```python
from build123d import *

# Parameters (mm, degrees)
SKETCH_1_R      = 1.1
EXTRUDE_1_DEPTH = 0.6
SKETCH_2_W      = 4.9
SKETCH_2_H      = 3.9
EXTRUDE_2_DEPTH = 1.75


with BuildPart() as part:
    # 草图1 → 凸台-拉伸1 (new body)
    with BuildSketch(Plane(origin=(0, 0, 0), x_dir=(1, 0, 0), z_dir=(0, 1, 0))):
        with BuildLine():
            Line((-4.123105626, 8), (4.123105626, 8))
            ThreePointArc((4.123105626, 8), (6.005155898, 6.703588789), (7.5, 4.974937186))
            Line((7.5, 4.974937186), (7.5, -4.974937186))
            ThreePointArc((7.5, -4.974937186), (6.005155898, -6.703588789), (4.123105626, -8))
            Line((4.123105626, -8), (-4.123105626, -8))
            ThreePointArc((-4.123105626, -8), (-6.005155898, -6.703588789), (-7.5, -4.974937186))
            Line((-7.5, -4.974937186), (-7.5, 4.974937186))
            ThreePointArc((-7.5, 4.974937186), (-6.005155898, 6.703588789), (-4.123105626, 8))
        make_face()
        with Locations((-6, 0)):
            Circle(SKETCH_1_R, mode=Mode.SUBTRACT)
        with Locations((6, 0)):
            Circle(SKETCH_1_R, mode=Mode.SUBTRACT)
    extrude(amount=EXTRUDE_1_DEPTH)

    # 草图2 → 凸台-拉伸2 (add)
    with BuildSketch(Plane(origin=(0, 0.6, 0), x_dir=(1, 0, 0), z_dir=(0, 1, 0))):
        Rectangle(SKETCH_2_W, SKETCH_2_H)
    extrude(amount=EXTRUDE_2_DEPTH)


solid = part.part
```
Source: CAD feature listing. Evaluate the final solid. Frame: model axes, mm. A direction names the side the tool comes from. Coordinates: 2 decimals unless noted, no trailing zeros. Write each loop counter-clockwise with the first axis right and the second up, starting at its lowest first coordinate (ties: lowest second). Pieces come first, ordered by that corner, then holes. Notation, with made-up numbers: (82.25, 85) -> (130.25, 85) arc R13 ccw to (130.25, 108) -> close; hole circle Ø1 at (80.5, -28). An arc over 180 degrees is marked (long way). Return JSON: item names as keys, results as strings. Group by question number.
1) Section query D-D, the plane x = -1.75. Return loops of the section in (y, z).
2) Mould query, pull axis X, two halves, no side actions, for faces 1 (the face through (0, 0, 0)), 2 (the face through (7.016, 0.296, 0.421)), 3 (the face through (-2.45, 1, 0)). Classes: +X half, -X half, draft (parallel to the pull), parting line (faces both ways), or undercut.
3) Section query C-C, the plane y = 0.3. Return loops of the section in (x, z).
4) Section query A-A, the plane z = 0. Return loops of the section in (x, y), plus the area to 3 significant figures.
5) Ray query, line 1 along X through (y, z) = (0.45, 0); line 2 along Y through (x, z) = (-0.5, -5.5); line 3 along Z through (x, y) = (6, 0.3). Return the intervals inside material, ascending.
6) Contact query for flat-ended pins moving along their axis: P1, Ø0.5, axis at x = 1, y = 1.5, coming from the +Z side; P2, Ø2, axis at x = 4.5, z = -3, coming from the +Y side; P3, Ø1, axis at x = 6, y = 1, coming from the +Z side. Output: stop coordinate, or through.
7) Section query B-B, the plane x = -6. Return loops of the section in (y, z), plus the area to 3 significant figures.
8) Set-up query: faces 4 (the face through (2.45, 1, 0)), 5 (the face through (0, 1, 1.95)), 6 (the face through (0, 1, -1.95)). Return all of +Z, -Z, +X, -X, +Y, -Y with unobstructed straight access to the full face (end or side cutting, diameter ignored); none if empty.
From the geometry:
{
 "1": {"outline": "(0, -8) -> (0.6, -8) -> (0.6, -1.95) -> (2.35, -1.95) -> (2.35, 1.95) -> (0.6, 1.95) -> (0.6, 8) -> (0, 8) -> close"},
 "2": {"face 1": "draft", "face 2": "undercut", "face 3": "-X half"},
 "3": {"outline": "(-7.5, -4.97) arc R9 ccw to (-4.12, -8) -> (4.12, -8) arc R9 ccw to (7.5, -4.97) -> (7.5, 4.97) arc R9 ccw to (4.12, 8) -> (-4.12, 8) arc R9 ccw to (-7.5, 4.97) -> close; hole circle Ø2.2 at (-6, 0); hole circle Ø2.2 at (6, 0)"},
 "4": {"outline": "(-7.5, 0) -> (-7.1, 0) -> (-7.1, 0.6) -> (-7.5, 0.6) -> close; (-4.9, 0) -> (4.9, 0) -> (4.9, 0.6) -> (2.45, 0.6) -> (2.45, 2.35) -> (-2.45, 2.35) -> (-2.45, 0.6) -> (-4.9, 0.6) -> close; (7.1, 0) -> (7.5, 0) -> (7.5, 0.6) -> (7.1, 0.6) -> close", "area": "14.9 mm²"},
 "5": {"line 1": "-7.5 to -7.1, -4.9 to 4.9, 7.1 to 7.5", "line 2": "0 to 0.6", "line 3": "-6.71 to -1.1, 1.1 to 6.71"},
 "6": {"P1": "z = 1.95", "P2": "y = 0.6", "P3": "z = 6.96"},
 "7": {"outline": "(0, -6.71) -> (0.6, -6.71) -> (0.6, -1.1) -> (0, -1.1) -> close; (0, 1.1) -> (0.6, 1.1) -> (0.6, 6.71) -> (0, 6.71) -> close", "area": "6.73 mm²"},
 "8": {"face 4": "+Z, -Z, +X, +Y", "face 5": "+Z, +X, -X, +Y", "face 6": "-Z, +X, -X, +Y"}
}
